Could you check a few things on this drawing? It's one solid part, dimensions in mm from its lowest x, y, z. A direction names the side the tool comes from. Give positions to 0.01 mm unless a question says otherwise; leave off trailing zeros. Loops run counter-clockwise (first coordinate to the right, second up) from the corner with the lowest first, then second, coordinate; pieces in that order, holes last. Notation, with made-up numbers: M 68,4 L 87,4 A28 ccw 87,36 Z; hole C -9,74.5 d4. An arc over 180 degrees is marked long. Write each question's results on one line, items separated by ' | '. Start each with the question number.
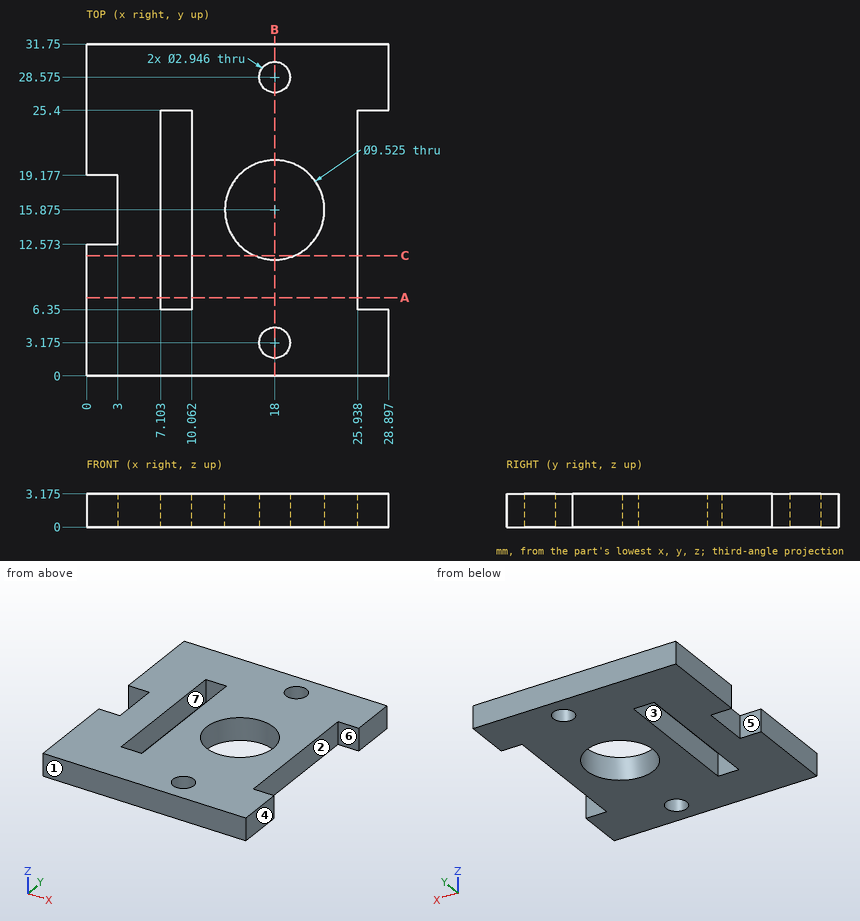
1) Thinking about a two-plate mould opening in Y: for the marked faces 1, 2, 3 and 4, which applies, pulls with the +Y half, pulls with the -Y half, needs draft (parallel to the pull), parting line crosses it, or undercut?
2) Please list where these lines run through material, in increasing order: line 1 (Y direction, x = 18, z = 2.2); line 2 (X direction, y = 21, z = 2.25); line 3 (X direction, y = 20, z = 2.6) (1 decimal). Write a range as from..to.
3) If we section it at C-C on y = 11.5: Write out the boundary of the cut face in (x, z) (1 decimal).
4) Which directions (+Z, -Z, +X, -X, +Y, -Y) give clear straight access to the entire face, cutting with the end or side of a thin tool? Please do the marked faces 5, 6 and 7.
5) If we section it at A-A on y = 7.5: Write out the boundary of the cut face in (x, z) (1 decimal).
6) I'm going to push flat-ended pins straight in: P1, Ø1.6, axis at y = 12, z = 1.5, coming from the -X side; P2, Ø7.5, axis at x = 18, y = 15.875, coming from the +Z side. Where does each tip first touch, or does it pass through?
7) If we section it at B-B on x = 18: State how many separate pieces and enclosed holes the cut face has.
Calculated:
1) face 1: pulls with the -Y half | face 2: undercut | face 3: undercut | face 4: needs draft
2) line 1: y = 0..1.7, 4.65..11.11, 20.64..27.1, 30.05..31.75 | line 2: x = 0..7.1, 10.06..25.94 | line 3: x = 0..7.1, 10.1..15.6, 20.4..25.9
3) outline: M 0,0 L 7.1,0 L 7.1,3.2 L 0,3.2 Z; M 10.1,0 L 16.1,0 L 16.1,3.2 L 10.1,3.2 Z; M 19.9,0 L 25.9,0 L 25.9,3.2 L 19.9,3.2 Z
4) face 5: +Z, -Z, -X | face 6: +Z, -Z, +X | face 7: +Z, -Z
5) outline: M 0,0 L 7.1,0 L 7.1,3.2 L 0,3.2 Z; M 10.1,0 L 25.9,0 L 25.9,3.2 L 10.1,3.2 Z
6) P1: stops at x = 0 | P2: passes through
7) separate pieces: 4 | enclosed holes: 0
